Part model, mm, in its own coordinate system. Round coordinates to 2 decimals unless told otherwise and drop trailing zeros. Order: outer loops, then holes, each group sorted by start corner. A loop starts at its lowest first (then second) coordinate and runs counter-clockwise, first axis right, second up. Notation, with made-up numbers: (-15, 22) -> (25, 22) arc R12 ccw to (25, 30) -> close; hole circle Ø1 at (-13.5, 23). An arc over 180 degrees is marked (long way). Return JSON: item names as keys, results as strings. Group by question number.
from build123d import *

# Parameters (mm, degrees)
SKETCH1_W                = 355
SKETCH1_H                = 100
BOSS_EXTRUDE1_DEPTH      = 2.54
SKETCH4_R                = 2.25
SKETCH4_R_2              = 30
CUT_EXTRUDE1_DEPTH       = 2.54
SKETCH5_W                = 100
SKETCH5_H                = 2.54
BOSS_EXTRUDE2_DEPTH      = 2.5
SKETCH6_W                = 100
SKETCH6_H                = 2.54
CUT_EXTRUDE2_DEPTH       = 2.5
SKETCH7_W                = 355
SKETCH7_H                = 2.54
BOSS_EXTRUDE3_DEPTH      = 60
SKETCH8_W                = 355
SKETCH8_H                = 2.54
BOSS_EXTRUDE4_DEPTH      = 60
M8_CLEARANCE_SLOT6_DEPTH = 2.54


# Read off the part's stored shape, not the designer's step: M8 Clearance Slot6
with BuildPart() as part:
    # Sketch1 → Boss-Extrude1 (new body)
    with BuildSketch(Plane(origin=(0, 0, 0), x_dir=(1, 0, 0), z_dir=(0, 1, 0))):
        with Locations((-6.378176495, -11.509617782)):
            Rectangle(SKETCH1_W, SKETCH1_H)
    extrude(amount=BOSS_EXTRUDE1_DEPTH)

    # Sketch4 → Cut-Extrude1 (cut)
    with BuildSketch(Plane(origin=(0, 0, 0), x_dir=(-1, 0, 0), z_dir=(0, -1, 0))):
        with Locations(Location((38.553176495, 20.665382218, 0), (0, 0, 90))):
            Circle(SKETCH4_R)
        with Locations(Location((-25.796823505, 20.665382218, 0), (0, 0, 90))):
            Circle(SKETCH4_R)
        with Locations(Location((-25.796823505, -43.684617782, 0), (0, 0, 90))):
            Circle(SKETCH4_R)
        with Locations(Location((38.553176495, -43.684617782, 0), (0, 0, 90))):
            Circle(SKETCH4_R)
        with Locations(Location((6.378176495, -11.509617782, 0), (0, 0, 90))):
            Circle(SKETCH4_R_2)
    extrude(amount=-CUT_EXTRUDE1_DEPTH, mode=Mode.SUBTRACT)

    # Sketch5 → Boss-Extrude2 (add)
    with BuildSketch(Plane.ZY.offset(183.878176495)):
        with Locations((11.509617782, 1.27)):
            Rectangle(SKETCH5_W, SKETCH5_H)
    extrude(amount=BOSS_EXTRUDE2_DEPTH)

    # Sketch6 → Cut-Extrude2 (cut)
    with BuildSketch(Plane(origin=(171.121823505, 0, 0), x_dir=(0, 0, -1), z_dir=(1, 0, 0))):
        with Locations((-11.509617782, 1.27)):
            Rectangle(SKETCH6_W, SKETCH6_H)
    extrude(amount=-CUT_EXTRUDE2_DEPTH, mode=Mode.SUBTRACT)

    # Sketch7 → Boss-Extrude3 (add)
    with BuildSketch(Plane(origin=(0, 0, -38.490382218), x_dir=(-1, 0, 0), z_dir=(0, 0, -1))):
        with Locations((8.878176495, 1.27)):
            Rectangle(SKETCH7_W, SKETCH7_H)
    extrude(amount=BOSS_EXTRUDE3_DEPTH)

    # Sketch8 → Boss-Extrude4 (add)
    with BuildSketch(Plane.XY.offset(61.509617782)):
        with Locations((-8.878176495, 1.27)):
            Rectangle(SKETCH8_W, SKETCH8_H)
    extrude(amount=BOSS_EXTRUDE4_DEPTH)

    # M8 Clearance Slot6 outline → M8 Clearance Slot6 (cut)
    with BuildSketch(Plane(origin=(0, 0, 0), x_dir=(1, 0, 0), z_dir=(0, 1, 0))):
        with BuildLine():
            Line((-169.579279891, 63.990382218), (-166.579279891, 63.990382218))
            ThreePointArc((-166.579279891, 63.990382218), (-162.079279891, 68.490382218), (-166.579279891, 72.990382218))
            Line((-166.579279891, 72.990382218), (-169.579279891, 72.990382218))
            ThreePointArc((-169.579279891, 72.990382218), (-174.079279891, 68.490382218), (-169.579279891, 63.990382218))
        make_face()
        with BuildLine():
            ThreePointArc((147.121823505, 72.990382218), (142.621823505, 68.490382218), (147.121823505, 63.990382218))
            Line((147.121823505, 63.990382218), (150.121823505, 63.990382218))
            ThreePointArc((150.121823505, 63.990382218), (154.621823505, 68.490382218), (150.121823505, 72.990382218))
            Line((150.121823505, 72.990382218), (147.121823505, 72.990382218))
        make_face()
        with BuildLine():
            Line((-169.579279891, -96.009617782), (-166.579279891, -96.009617782))
            ThreePointArc((-166.579279891, -96.009617782), (-162.079279891, -91.509617782), (-166.579279891, -87.009617782))
            Line((-166.579279891, -87.009617782), (-169.579279891, -87.009617782))
            ThreePointArc((-169.579279891, -87.009617782), (-174.079279891, -91.509617782), (-169.579279891, -96.009617782))
        make_face()
        with BuildLine():
            ThreePointArc((150.121823505, -96.009617782), (154.621823505, -91.509617782), (150.121823505, -87.009617782))
            Line((150.121823505, -87.009617782), (147.121823505, -87.009617782))
            ThreePointArc((147.121823505, -87.009617782), (142.621823505, -91.509617782), (147.121823505, -96.009617782))
            Line((147.121823505, -96.009617782), (150.121823505, -96.009617782))
        make_face()
        with BuildLine():
            ThreePointArc((-166.579279891, -16.009617782), (-162.079279891, -11.509617782), (-166.579279891, -7.009617782))
            Line((-166.579279891, -7.009617782), (-169.579279891, -7.009617782))
            ThreePointArc((-169.579279891, -7.009617782), (-174.079279891, -11.509617782), (-169.579279891, -16.009617782))
            Line((-169.579279891, -16.009617782), (-166.579279891, -16.009617782))
        make_face()
        with BuildLine():
            ThreePointArc((150.121823505, -16.009617782), (154.621823505, -11.509617782), (150.121823505, -7.009617782))
            Line((150.121823505, -7.009617782), (147.121823505, -7.009617782))
            ThreePointArc((147.121823505, -7.009617782), (142.621823505, -11.509617782), (147.121823505, -16.009617782))
            Line((147.121823505, -16.009617782), (150.121823505, -16.009617782))
        make_face()
    extrude(amount=M8_CLEARANCE_SLOT6_DEPTH, mode=Mode.SUBTRACT)


solid = part.part
(1) Saw through at B-B, the plane y = 1.95. State how many separate pieces and enclosed holes the cut face has, and give its area (3 significant figures).
(2) Saw through at A-A, the plane z = -2. List the corners of the cut face in (x, y).
(3) Mould opens along X. For faces 1 (the flat face through (28, 0, 10)), 2 (the cylindrical face through (-17.87, 1.25, -16.2)) say: pulls with the +X half, pulls with the -X half, needs draft (parallel to the pull), parting line crosses it, or undercut.
(4) Pin check, flat tip, straight feed: P1, Ø3.5, axis at x = -38.55, z = 43.68, coming from the +Y side. Stop position of the tip, or through.
(5) Probe L1, parallel to Z at x = 147.5, y = 2.2; L2, parallel to X at y = 2.35, z = 43; L3, parallel to X at y = 2.1, z = 7.5. List the from-to ranges inside material, lowest first. Write a range as [from, to].
Results are:
{
 "1": {"separate pieces": "1", "enclosed holes": "11", "area": "74,700 mm^2"},
 "2": {"outline": "(-186.38, 0) -> (-33.16, 0) -> (-33.16, 2.54) -> (-186.38, 2.54) -> close; (20.41, 0) -> (168.62, 0) -> (168.62, 2.54) -> (20.41, 2.54) -> close"},
 "3": {"face 1": "needs draft", "face 2": "undercut"},
 "4": {"P1": "passes through"},
 "5": {"L1": "z = [-98.49, -72.99], [-63.99, 7.01], [16.01, 87.01], [96.01, 121.51]", "L2": "x = [-186.38, -40.7], [-36.41, 23.65], [27.94, 168.62]", "L3": "x = [-186.38, -171.62], [-164.54, -36.11], [23.35, 145.08], [152.16, 168.62]"}
}
